Source: CAD feature listing. Evaluate the final solid. Frame: model axes, mm. Face numbers are marked on the shaded views. A direction names the side the tool comes from. Give positions to 0.01 mm unless a question says otherwise; leave off trailing zeros. Order: outer loops, then holes, each group sorted by start corner. A loop starts at its lowest first (then second) coordinate and runs counter-clockwise, first axis right, second up.
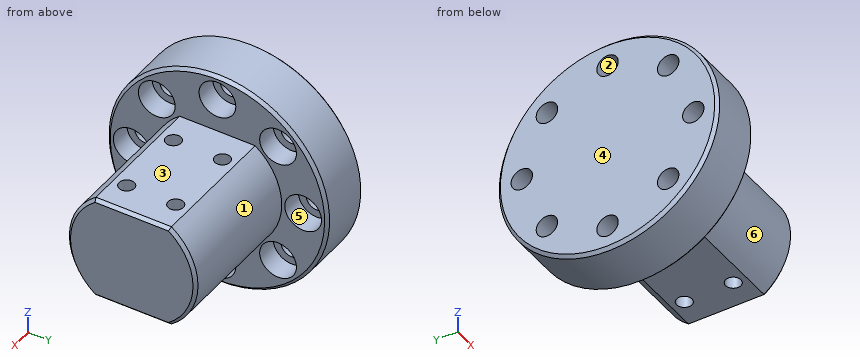
```python
from build123d import *

# Parameters (mm, degrees)
SKETCH1_R           = 18
BOSS_EXTRUDE1_DEPTH = 9
SKETCH2_R           = 10.5
BOSS_EXTRUDE2_DEPTH = 22
SKETCH3_R           = 1.75
CUT_EXTRUDE2_DEPTH  = 34.645207683
SKETCH3_3_R         = 3
SKETCH3_3_R_2       = 1.75
CUT_EXTRUDE3_DEPTH  = 3.5
CIRPATTERN1_COUNT   = 8
CHAMFER1_SIZE       = 0.5
CUT_EXTRUDE4_DEPTH  = 34.645207683
M3_TAPPED_HOLE1_D   = 2.5
CHAMFER2_SIZE       = 0.5


with BuildPart() as part:
    # Sketch1 → Boss-Extrude1 (new body)
    with BuildSketch(Plane(origin=(0, 0, 0), x_dir=(0, 0, -1), z_dir=(1, 0, 0))):
        Circle(SKETCH1_R)
    extrude(amount=BOSS_EXTRUDE1_DEPTH)

    # Sketch2 → Boss-Extrude2 (add)
    with BuildSketch(Plane(origin=(9, 0, 0), x_dir=(0, 0, -1), z_dir=(1, 0, 0))):
        Circle(SKETCH2_R)
    extrude(amount=BOSS_EXTRUDE2_DEPTH)

    # Sketch3 → Cut-Extrude2 (cut, through all)
    with BuildSketch(Plane(origin=(9, 0, 0), x_dir=(0, 0, -1), z_dir=(1, 0, 0))):
        with Locations((0, 14)):
            Circle(SKETCH3_R)
    cut_extrude2 = extrude(amount=-CUT_EXTRUDE2_DEPTH, mode=Mode.SUBTRACT)

    # Sketch3_3 → Cut-Extrude3 (cut)
    with BuildSketch(Plane(origin=(9, 0, 0), x_dir=(0, 0, -1), z_dir=(1, 0, 0))):
        with Locations((0, 14)):
            Circle(SKETCH3_3_R)
        with Locations((0, 14)):
            Circle(SKETCH3_3_R_2, mode=Mode.SUBTRACT)
    cut_extrude3 = extrude(amount=-CUT_EXTRUDE3_DEPTH, mode=Mode.SUBTRACT)

    # CirPattern1: Cut-Extrude2, Cut-Extrude3 ×8 about axis
    cirpattern1_axis = Axis((0, 0, 0), (1, 0, 0))
    add([cut_extrude2.rotate(cirpattern1_axis, i * 360 / CIRPATTERN1_COUNT) for i in range(1, CIRPATTERN1_COUNT)], mode=Mode.SUBTRACT)
    add([cut_extrude3.rotate(cirpattern1_axis, i * 360 / CIRPATTERN1_COUNT) for i in range(1, CIRPATTERN1_COUNT)], mode=Mode.SUBTRACT)

    # Chamfer1
    chamfer1_edges = [part.edges().sort_by_distance(p)[0] for p in [
        (0, 0, 18),
        (9, 0, 18),
    ]]
    chamfer(chamfer1_edges, length=CHAMFER1_SIZE)

    # Sketch4 → Cut-Extrude4 (cut, through all)
    with BuildSketch(Plane(origin=(9, 0, 0), x_dir=(0, 0, -1), z_dir=(1, 0, 0))):
        with BuildLine():
            Line((-8.5, 4), (-8.5, 6.164414003))
            ThreePointArc((-8.5, 6.164414003), (-10.5, 0), (-8.5, -6.164414003))
            Line((-8.5, -6.164414003), (-8.5, -4))
            Line((-8.5, -4), (-8.5, 4))
        make_face()
        with BuildLine():
            ThreePointArc((10.5, 0), (9.987492178, 3.240370349), (8.5, 6.164414003))
            Line((8.5, 6.164414003), (8.5, -6.164414003))
            ThreePointArc((8.5, -6.164414003), (9.987492178, -3.240370349), (10.5, 0))
        make_face()
    extrude(amount=CUT_EXTRUDE4_DEPTH, mode=Mode.SUBTRACT)

    # M3 Tapped Hole1 (through all)
    with Locations(Plane(origin=(14, 4, 8.5), x_dir=(1, 0, 0), z_dir=(0, 0, 1))):
        with Locations((0, 0), (12, 0), (0, -8), (12, -8)):
            Hole(M3_TAPPED_HOLE1_D / 2)

    # Chamfer2
    chamfer2_edges = [part.edges().sort_by_distance(p)[0] for p in [
        (31, -10.5, 0),
        (31, 0, 8.5),
        (31, 0, -8.5),
        (31, 10.5, 0),
    ]]
    chamfer(chamfer2_edges, length=CHAMFER2_SIZE)


solid = part.part
```
1) Reachability of the marked faces 4, 5 and 6 from +Z, -Z, +X, -X, +Y, -Y: full face, straight path, thin tool, end or side. Return the list, or none.
Report:
face 4: +Z, -Z, -X, +Y, -Y
face 5: +X
face 6: +X, -Y
2) Section query A-A, the plane y = 0. Count the separate pieces of the cut face and the enclosed holes in it, and give its area (3 significant figures).
Report:
separate pieces: 3
enclosed holes: 0
area: 617 mm2
3) Section query B-B, the plane x = 26. Return the cut outline in (y, z), and give its area (3 significant figures).
Report:
outline: (-6.16, -8.5) - (-5.25, -8.5) - (-5.25, 8.5) - (-6.16, 8.5) arc R10.5 ccw to start; (-2.75, -8.5) - (2.75, -8.5) - (2.75, 8.5) - (-2.75, 8.5) - close; (5.25, -8.5) - (6.16, -8.5) arc R10.5 ccw to (6.16, 8.5) - (5.25, 8.5) - close
area: 228 mm2
4) Material intervals for L1, parallel to Y at x = 3.75, z = 0; L2, parallel to Y at x = 14, z = 0; L3, parallel to X at y = 5, z = 1.5, sorted ascending.
Report:
L1: y = -18 to -15.75, -12.25 to 12.25, 15.75 to 18
L2: y = -10.5 to -5.25, -2.75 to 2.75, 5.25 to 10.5
L3: x = 0 to 13.25, 14.75 to 25.25, 26.75 to 31
5) Draft query along Z for the marked faces 1, 2 and 3. Return one class per face: +Z half, -Z half, draft (parallel to the pull), parting line (faces both ways), or undercut.
Report:
face 1: parting line
face 2: undercut
face 3: +Z half
6) Pin query (flat end, axial travel): pin 1 (1.5 mm diameter, centred on y = 9.5, z = -3.5, fed in from -X); pin 2 (3 mm diameter, centred on x = 14, y = 4, fed in from +Z); pin 3 (6.5 mm diameter, centred on y = 8.5, z = 10.5, fed in from +X); pin 4 (4 mm diameter, centred on x = 11.5, z = 14, fed in from -Y). Return the tip coordinate at first contact, or that it passes through.
Report:
pin 1: stops at x = 0
pin 2: stops at z = 8.5
pin 3: stops at x = 30.74
pin 4: passes through
